from build123d import *

# Parameters (mm, degrees)
SKETCH1_R           = 254
BOSS_EXTRUDE3_DEPTH = 254
BOSS_EXTRUDE4_DEPTH = 1016
BOSS_EXTRUDE5_START = 762
SKETCH1_9_W         = 508
SKETCH1_9_H         = 254
BOSS_EXTRUDE5_DEPTH = 254


with BuildPart() as part:
    # Sketch1 → Boss-Extrude3 (new body)
    with BuildSketch(Plane.XY):
        with BuildLine():
            Line((0, 0), (1524, 0))
            Line((1524, 0), (1524, 508))
            ThreePointArc((1524, 508), (1016, 1016), (508, 508))
            Line((508, 508), (0, 508))
            Line((0, 508), (0, 0))
        make_face()
        with Locations((1016, 508)):
            Circle(SKETCH1_R, mode=Mode.SUBTRACT)
    extrude(amount=BOSS_EXTRUDE3_DEPTH)

    # Sketch1_8 → Boss-Extrude4 (add)
    with BuildSketch(Plane.XY):
        Polygon((0, 254), (0, 0), (1524, 0), (1524, 254), (1016, 254), (508, 254), align=None)
    extrude(amount=BOSS_EXTRUDE4_DEPTH)

    # Sketch1_9 → Boss-Extrude5 (add)
    with BuildSketch(Plane.XY.offset(BOSS_EXTRUDE5_START)):
        with BuildLine():
            Line((0, 762), (0, 508))
            Line((0, 508), (508, 508))
            ThreePointArc((508, 508), (328.394877579, 582.394877579), (254, 762))
            Line((254, 762), (0, 762))
        make_face()
        with Locations((254, 381)):
            Rectangle(SKETCH1_9_W, SKETCH1_9_H)
    extrude(amount=BOSS_EXTRUDE5_DEPTH)


solid = part.part
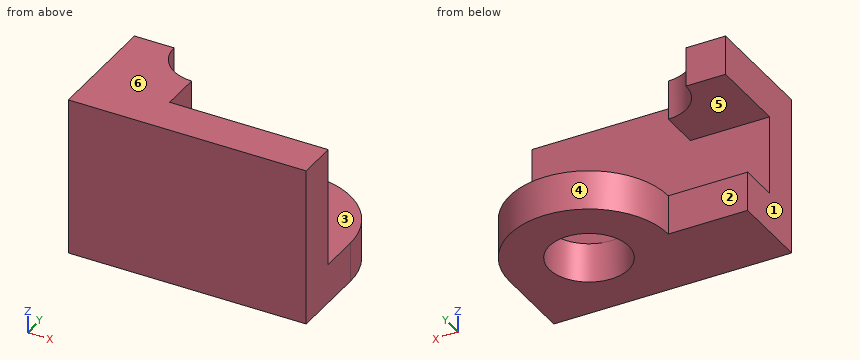
The listing builds one solid part. Answer for the finished solid, in the listing's coordinates (mm). Face numbers are marked on the shaded views. A direction names the side the tool comes from. Round coordinates to 2 decimals unless told otherwise and drop trailing zeros. Loops run counter-clockwise (first coordinate to the right, second up) from the corner with the lowest first, then second, coordinate; pieces in that order, holes last. Notation, with made-up numbers: M 51,63.25 L 106,63.25 A27 ccw 106,95.25 Z; hole C -31.5,34 d9. An arc over 180 degrees is marked long. Return JSON: item names as keys, results as strings.
Q1. Find section B-B, the plane y = 449.5. Determine the outline of the cut face in (x, z), plus the area to 3 significant figures.
Results list:
{"outline": "M 0,0 L 768.83,0 L 768.83,254 L 0,254 Z; M 0,762 L 508,762 L 508,1016 L 0,1016 Z; M 1263.17,0 L 1524,0 L 1524,254 L 1263.17,254 Z", "area": "391,000 mm2"}
Q2. The mould has two halves that part along Z. Classify the marked faces 4, 5 and 6: released by +Z, released by -Z, zero draft, split by the parting line, or undercut.
Results list:
{"face 4": "zero draft", "face 5": "undercut", "face 6": "released by +Z"}
Q3. Find section D-D, the plane x = 473. Determine the outline of the cut face in (y, z).
Results list:
{"outline": "M 0,0 L 508,0 L 508,254 L 254,254 L 254,762 L 510.42,762 L 510.42,1016 L 0,1016 Z"}
Q4. Find section A-A, the plane x = 798. Determine the outline of the cut face in (y, z), plus the area to 3 significant figures.
Results list:
{"outline": "M 0,0 L 377.65,0 L 377.65,254 L 254,254 L 254,1016 L 0,1016 Z; M 638.35,0 L 966.85,0 L 966.85,254 L 638.35,254 Z", "area": "373,000 mm2"}
Q5. Each of these flat-tipped pins is pushed along its axis until it touches: pin 1 Ø1.5 at (y, z) = (672.5, 154) entering from -X; pin 2 Ø6 at (x, z) = (239, 663.5) entering from +Y. Where does it stop, or does it pass through?
Results list:
{"pin 1": "stops at x = 535.12", "pin 2": "stops at y = 254"}
Q6. Find the intervals of material crossed by line 1 along Y through (x, z) = (1016, 191); line 2 along Y through (x, z) = (1254.5, 342), in increasing order. Write a range as from..to.
Results list:
{"line 1": "y = 0..254, 762..1016", "line 2": "y = 0..254"}
Q7. Find section C-C, the plane z = 801.5. Determine the outline of the cut face in (x, y).
Results list:
{"outline": "M 0,0 L 1524,0 L 1524,254 L 508,254 L 508,508 A254 cw 254,762 L 0,762 Z"}
Q8. Which of the six approach directions +Z, -Z, +X, -X, +Y, -Y give full straight-line access (tool end or side, diameter ignored) to the marked faces 1, 2 and 3?
Results list:
{"face 1": "+Z, -Z, -X, +Y, -Y", "face 2": "-Z, -X, +Y", "face 3": "+X, -X, +Y"}
